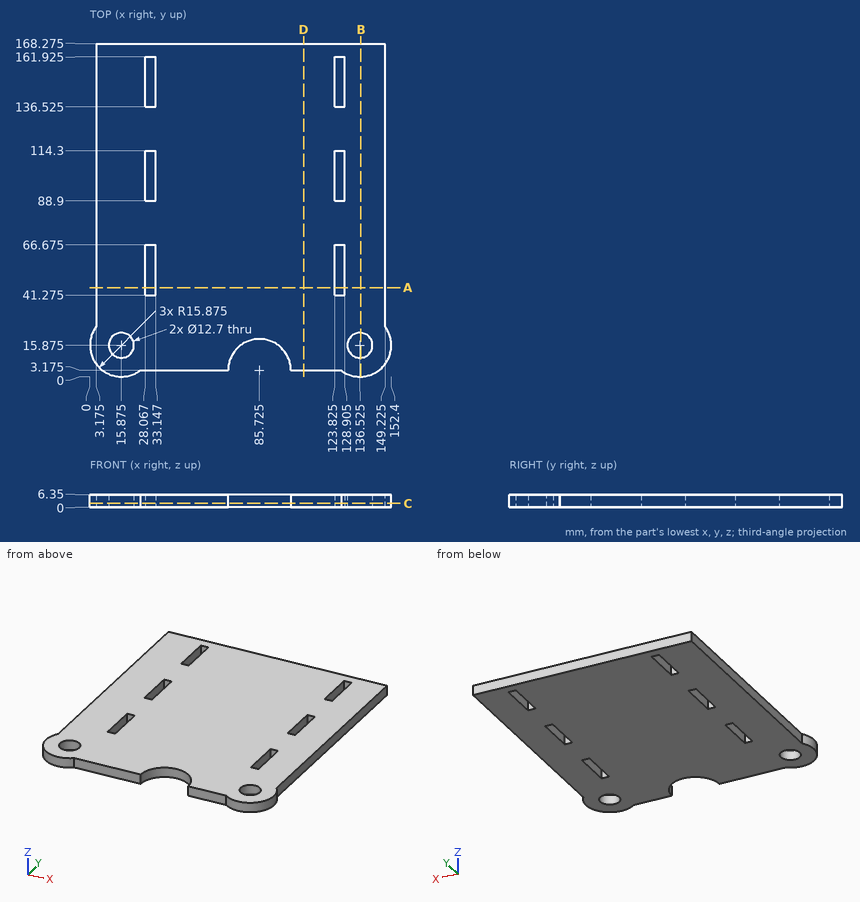
For this review, use the dimensioned drawing (mm, ordinates from the lowest corner) and the shaded views. Coordinates: 2 decimals unless noted, no trailing zeros. Loops run counter-clockwise (first coordinate to the right, second up) from the corner with the lowest first, then second, coordinate; pieces in that order, holes last. Notation, with made-up numbers: (3.25, -27.75) -> (10.25, -27.75) arc R30 cw to (10.25, 4.25) -> close; hole circle Ø5 at (-25.75, -9.5). An arc over 180 degrees is marked (long way). Return JSON: item names as keys, results as strings. Group by question number.
(1) Consider section B-B, the plane x = 137. Give the boundary of the cut face in (y, z) (3 decimals).
(2) For pin 1 Ø11.5 at (x, y) = (136.525, 15.875) entering from +Z; pin 2 Ø1.9 at (y, z) = (107, 4) entering from +X (3 decimals); pin 3 Ø3 at (y, z) = (97, 2.5) entering from -X (3 decimals), all flat-tipped, find the tip position at first contact; note any pin that passes through.
(3) To check wall thickness, follow L1, parallel to X at y = 48.5, z = 2.75 (3 decimals); L2, parallel to Y at x = 125, z = 3 (3 decimals); L3, parallel to Y at x = 57, z = 3.25 (3 decimals). State the ranges of each line that lie inside material, in increasing order.
(4) Consider section D-D, the plane x = 108. Give the boundary of the cut face in (y, z) (3 decimals), plus the area to 3 significant figures.
(5) Consider section A-A, the plane y = 45. Give the boundary of the cut face in (x, z) (3 decimals), plus the area to 3 significant figures.
(6) Consider section C-C, the plane z = 2. Count the separate pieces of the cut face and the enclosed holes in it, plus the area to 3 significant figures.
Results below:
{
 "1": {"outline": "(0.007, 0) -> (9.543, 0) -> (9.543, 6.35) -> (0.007, 6.35) -> close; (22.207, 0) -> (168.275, 0) -> (168.275, 6.35) -> (22.207, 6.35) -> close"},
 "2": {"pin 1": "passes through", "pin 2": "stops at x = 149.225", "pin 3": "stops at x = 3.175"},
 "3": {"L1": "x = 3.175 to 28.067, 33.147 to 123.825, 128.905 to 149.225", "L2": "y = 3.175 to 41.275, 66.675 to 88.9, 114.3 to 136.525, 161.925 to 168.275", "L3": "y = 3.175 to 168.275"},
 "4": {"outline": "(3.175, 0) -> (168.275, 0) -> (168.275, 6.35) -> (3.175, 6.35) -> close", "area": "1,050 mm2"},
 "5": {"outline": "(3.175, 0) -> (28.067, 0) -> (28.067, 6.35) -> (3.175, 6.35) -> close; (33.147, 0) -> (123.825, 0) -> (123.825, 6.35) -> (33.147, 6.35) -> close; (128.905, 0) -> (149.225, 0) -> (149.225, 6.35) -> (128.905, 6.35) -> close", "area": "863 mm2"},
 "6": {"separate pieces": "1", "enclosed holes": "8", "area": "22,800 mm2"}
}
